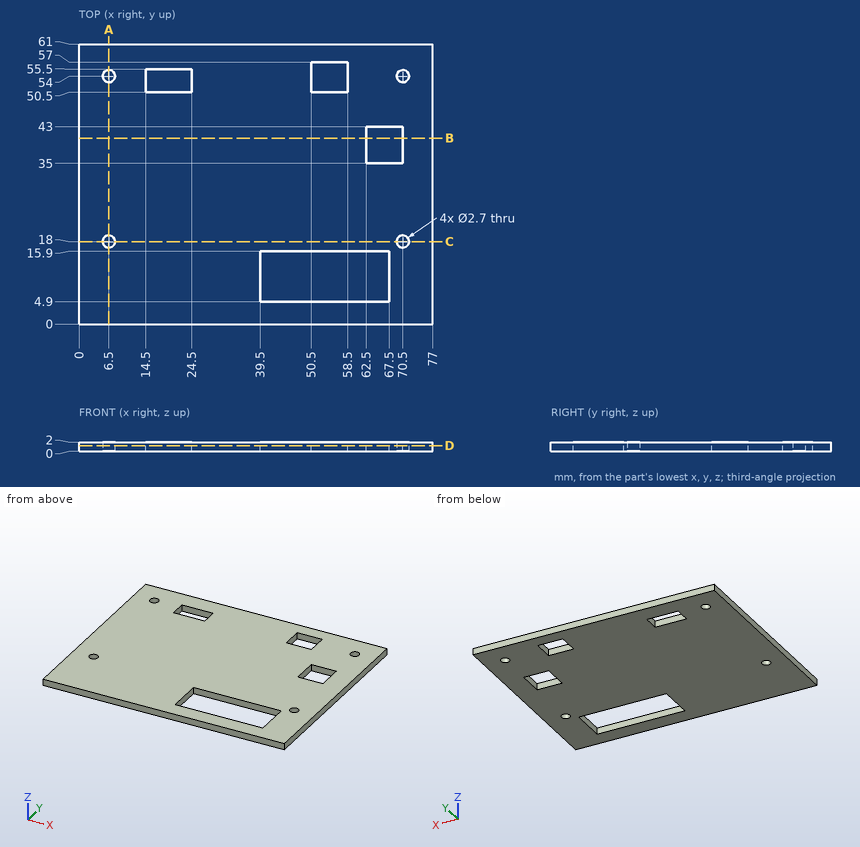
Print and shaded views of the part. All mm, measured from the part's lowest x, y and z. Coordinates: 2 decimals unless noted, no trailing zeros. Loops run counter-clockwise (first coordinate to the right, second up) from the corner with the lowest first, then second, coordinate; pieces in that order, holes last. Notation, with made-up numbers: (-24, 65.5) - (33, 65.5) arc R29 ccw to (33, 103.5) - close; hole circle Ø10 at (-16.5, -35.75). An arc over 180 degrees is marked (long way). Use one line per item in the form item = value. Start each with the question number.
1) Band-saw the part on D-D (z = 1.25). State how many separate pieces and enclosed holes the cut face has, and give its area (3 significant figures).
2) Band-saw the part on A-A (x = 6.5). Give the cut face in (y, z).
3) Band-saw the part on C-C (y = 18). Give the cut face in (x, z), and give its area (3 significant figures).
4) Drill centre lines: L1, parallel to X at y = 54, z = 0.95; L2, parallel to X at y = 18, z = 0.8; L3, parallel to Y at x = 55, z = 0.15. Where is each one in solid material? Low to high. Write a range as from..to.
5) Band-saw the part on B-B (y = 40.5). Give the cut face in (x, z), and give its area (3 significant figures).
Check values:
q1.separate_pieces = 1
q1.enclosed_holes = 8
q1.area = 4,200 mm2
q2.outline = (0, 0) - (16.65, 0) - (16.65, 2) - (0, 2) - close; (19.35, 0) - (52.65, 0) - (52.65, 2) - (19.35, 2) - close; (55.35, 0) - (61, 0) - (61, 2) - (55.35, 2) - close
q3.outline = (0, 0) - (5.15, 0) - (5.15, 2) - (0, 2) - close; (7.85, 0) - (69.15, 0) - (69.15, 2) - (7.85, 2) - close; (71.85, 0) - (77, 0) - (77, 2) - (71.85, 2) - close
q3.area = 143 mm2
q4.L1 = 0..5.15, 7.85..14.5, 24.5..50.5, 58.5..69.15, 71.85..77
q4.L2 = 0..5.15, 7.85..69.15, 71.85..77
q4.L3 = 0..4.9, 15.9..50.5, 57..61
q5.outline = (0, 0) - (62.5, 0) - (62.5, 2) - (0, 2) - close; (70.5, 0) - (77, 0) - (77, 2) - (70.5, 2) - close
q5.area = 138 mm2
